Input: part model. Units: mm. Frame: model coordinates. Coordinates: 2 decimals unless noted, no trailing zeros. Write each loop counter-clockwise with the first axis right and the second up, starting at its lowest first coordinate (ties: lowest second). Pieces come first, ordered by that corner, then holes. Notation, with made-up numbers: M 41,69 L 70,69 A12 ccw 70,73 Z; hole C -32.5,-12 d6. An arc over 180 degrees is marked long. Use one line per item in the form item = value.
Autodesk Inventor part; units mm, degrees
ref_plane "Work Plane1" through (0, 0, 2.5241) normal (0, 0, 1) x (1, 0, 0)
ref_plane "YZ Plane" through (0, 0, 0) normal (1, 0, 0) x (0, 1, 0)
ref_plane "XZ Plane" through (0, 0, 0) normal (0, 1, 0) x (-1, 0, 0)
ref_plane "Work Plane1" through (0, 0, 2.5241) normal (0, 0, 1) x (1, 0, 0)
sketch "Sketch1" plane through (0, 0, 2.5241) normal (0, 0, 1) x (1, 0, 0)
  line L0 (16, 228) -> (4, 228) construction
  line L1 (4, 148) -> (-8, 148) construction
  line L2 (4, 228) -> (-4.0164, 228)
  line L3 (-4.0164, 228) -> (-4.0164, 148)
  line L4 (-4.0164, 148) -> (4, 148)
  line L5 (4, 148) -> (4, 228)
  point P0 (0, 0)
extrude "Extrusion1" add sketch "Sketch1" along normal blind 17.78
sketch "Sketch2" plane through (-4.0164, 148, 2.5241) normal (0, -1, 0) x (1, 0, 0)
  line L0 (0, 17.78) -> (8.0164, 17.78) construction
  line L1 (0, 0) -> (0, 17.78) construction
  line L2 (0, 0) -> (0, 17.78)
  line L3 (8.0164, 17.78) -> (0, 17.78)
  line L4 (0, 0) -> (0, 17.78)
  line L5 (0, 17.78) -> (5.969, 17.78)
  line L6 (5.969, 17.78) -> (0, 0)
  point P0 (4.0164, -2.5241)
  dimension "d2" = 5.969
extrude "Extrusion2" cut sketch "Sketch2" against normal up to surface (80 mm away)
sketch "Sketch3" plane through (0, 0, 2.5241) normal (0, 0, -1) x (-1, 0, 0)
  circle A0 centre (0, 220) radius 2 construction
  circle A1 centre (0, 156) radius 2 construction
  circle A2 centre (0, 188) radius 2 construction
  point P0 (0, 0)
hole "Hole1" at (0, 220, 2.5241) at (0, 188, 2.5241) at (0, 156, 2.5241) direction (0, 0, 1) diameter 3.937 depth 6.35
properties part number "EjectionRamp"
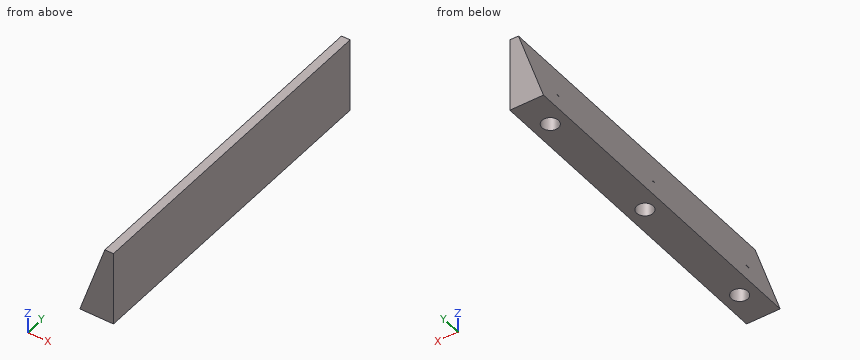
(1) First-contact query: pin 1 Ø4 at (x, y) = (0.5, 189) entering from -Z; pin 2 Ø3 at (y, z) = (217.5, 5) entering from -X; pin 3 Ø3 at (x, y) = (0, 156) entering from -Z; pin 4 Ø1.5 at (y, z) = (159.5, 13.5) entering from -X. Flat tips, straight axial feed; report the tip coordinate or a pass-through.
Computed:
pin_1 = 2.52
pin_2 = -3.69
pin_3 = 8.87
pin_4 = -0.58
(2) Line query: probe 1 along Y at (x, z) = (0, 7); probe 2 along Y at (x, z) = (0.75, 7); probe 3 along X at (y, z) = (156, 4.75). Output: solid intervals per line, ascending.
Computed:
probe_1 = 148 to 154.03, 157.97 to 186.03, 189.97 to 218.03, 221.97 to 228
probe_2 = 148 to 154.18, 157.82 to 186.18, 189.82 to 218.18, 221.82 to 228
probe_3 = -3.27 to -1.97, 1.97 to 4
(3) Section query C-C on z = 12.75. Return the cut outline in (x, y).
Computed:
outline = M -0.58,148 L 4,148 L 4,228 L -0.58,228 Z
(4) Section query A-A on y = 160. Return the cut outline in (x, z), plus the area to 3 significant figures.
Computed:
outline = M -4.02,2.52 L 4,2.52 L 4,20.3 L 1.95,20.3 Z
area = 89.5 mm^2
(5) Section query B-B on x = 0. Return the cut outline in (y, z), plus the area to 3 significant figures.
Computed:
outline = M 148,2.52 L 154.03,2.52 L 154.03,8.87 L 157.97,8.87 L 157.97,2.52 L 186.03,2.52 L 186.03,8.87 L 189.97,8.87 L 189.97,2.52 L 218.03,2.52 L 218.03,8.87 L 221.97,8.87 L 221.97,2.52 L 228,2.52 L 228,14.49 L 148,14.49 Z
area = 882 mm^2
